Autodesk Fusion 360 part; units mm, degrees
sketch "Sketch1" plane through (0, 0, 0) normal (0, 0, 1) x (1, 0, 0)
  circle A0 centre (0, 0) radius 11
  circle A1 centre (0, 0) radius 4
  dimension "d1_4" = 22
  dimension "d2_4" = 8
extrude "Extrude1" add sketch "Sketch1" along normal blind 3.8
sketch "Sketch2" plane through (0, 0, 3.8) normal (0, 0, 1) x (-1, 0, 0)
  circle A0 centre (0, 0) radius 4
  circle A1 centre (0, 0) radius 11
  circle A2 centre (0, 0) radius 5
  dimension "d5_1" = 10
extrude "Extrude2" add sketch "Sketch2" along normal blind 5 contours A2
sketch "Sketch3" plane through (0, 0, 0) normal (0, 0, -1) x (1, 0, 0)
  circle A0 centre (0, 0) radius 4
  circle A1 centre (0, 0) radius 11
  circle A2 centre (0, 0) radius 5
  dimension "d8_1" = 10
extrude "Extrude3" add sketch "Sketch3" along normal blind 1.7 contours A2
sketch "Sketch4" plane through (0, 0, 3.8) normal (0, 0, 1) x (-1, 0, 0)
  circle A0 centre (0, 0) radius 5
  circle A1 centre (0, 0) radius 11
  circle A2 centre (0, 0) radius 8 construction
  circle A3 centre (0, 8) radius 1.4
  line L0 (0, 0) -> (-15, 0) construction
  circle A4 centre (-8, 0) radius 1.4
  circle A5 centre (8, 0) radius 1.4
  circle A6 centre (0, -8) radius 1.4
  dimension "d11_1" = 16
  dimension "d12_1" = 2.8
  dimension "d13_1" = 2.8
  dimension "d14_1" = 2.8
  dimension "d15_1" = 2.8
hole "Hole1" at (8, 0, 3.8) at (0, 8, 3.8) at (0, -8, 3.8) at (-8, 0, 3.8) direction (0, 0, -1) diameter 2.529 depth 3 tip angle 118
thread "Thread2" thread offset 0 thread length 10
equation "d9_1 = 10.5 mm - 8.8 mm"
Input: part model. Units: mm. Frame: model coordinates. A direction names the side the tool comes from. Give positions to 0.01 mm unless a question says otherwise; leave off trailing zeros. Order: outer loops, then holes, each group sorted by start corner. A loop starts at its lowest first (then second) coordinate and runs counter-clockwise, first axis right, second up.
1. Pin query (flat end, axial travel): pin 1 (2 mm diameter, centred on y = 2, z = 5.5, fed in from -X); pin 2 (6 mm diameter, centred on x = 7.5, z = 2, fed in from -Y); pin 3 (3.5 mm diameter, centred on x = 0, y = -8, fed in from -Z). Return the tip coordinate at first contact, or that it passes through.
Derived:
pin 1: stops at x = -4.9
pin 2: stops at y = -10.04
pin 3: stops at z = 0
2. Section A-A on x = 2.5. Return the cut outline in (y, z), and give its area (3 significant figures).
Derived:
outline: (-10.71, 0) - (-4.33, 0) - (-4.33, -1.7) - (-3.12, -1.7) - (-3.12, 8.8) - (-4.33, 8.8) - (-4.33, 3.8) - (-10.71, 3.8) - close; (3.12, -1.7) - (4.33, -1.7) - (4.33, 0) - (10.71, 0) - (10.71, 3.8) - (4.33, 3.8) - (4.33, 8.8) - (3.12, 8.8) - close
area: 73.9 mm2
3. Section B-B on z = 2.75. Return the cut outline in (x, y).
Derived:
outline: circle Ø22 at (0, 0); hole circle Ø2.53 at (-8, 0); hole circle Ø8 at (0, 0); hole circle Ø2.53 at (0, -8); hole circle Ø2.53 at (0, 8); hole circle Ø2.53 at (8, 0)
4. Section C-C on z = 6.5. Return the cut outline in (x, y).
Derived:
outline: circle Ø10 at (0, 0); hole circle Ø8 at (0, 0)
5. Mould query, pull axis Y, two halves, no side actions, for faces 1 (the cylindrical face through (1.08, -4.88, 6.26)), 2 (the flat face through (2, -5, 0)), 3 (the conical face through (0.01, -7.781, 0.172)). Classes: released by +Y, released by -Y, zero draft, split by the parting line, or undercut.
Derived:
face 1: split by the parting line
face 2: zero draft
face 3: undercut
6. Section D-D on x = -4.5. Return the cut outline in (y, z), and give its area (3 significant figures).
Derived:
outline: (-10.04, 0) - (-2.18, 0) - (-2.18, -1.7) - (2.18, -1.7) - (2.18, 0) - (10.04, 0) - (10.04, 3.8) - (2.18, 3.8) - (2.18, 8.8) - (-2.18, 8.8) - (-2.18, 3.8) - (-10.04, 3.8) - close
area: 105 mm2
7. Reachability of faces 4 (the cylindrical face through (-0.056, -6.737, 2.279)), 5 (the cylindrical face through (-1.08, -4.88, -0.84)), 6 (the cylindrical face through (-2.38, 10.74, 1.87)) from +Z, -Z, +X, -X, +Y, -Y: full face, straight path, thin tool, end or side. Return the list, or none.
Derived:
face 4: +Z
face 5: -Z
face 6: +Z, -Z
8. Material intervals for L1, parallel to Y at x = 0, z = 2.3; L2, parallel to X at y = 0, z = 6.5, sorted ascending.
Derived:
L1: y = -11 to -9.26, -6.74 to -4, 4 to 6.74, 9.26 to 11
L2: x = -5 to -4, 4 to 5
